Can you work these out from the model? Positions are in its coordinate system, mm. A direction names the side the tool comes from. Coordinates: 2 decimals unless noted, no trailing zeros. Order: outer loops, then holes, each group sorted by start corner. A loop starts at its lowest first (then second) coordinate and runs counter-clockwise, first axis right, second up. Notation, with made-up numbers: (16.25, -8) - (49.25, -8) arc R21 cw to (49.25, 2) - close; hole circle Ø10 at (6, -29.75). An arc over 180 degrees is marked (long way). Return JSON: item names as keys, results as strings. Group by question number.
1) If we mould it in two halves opening along X, with no side actions, what happens to faces 4 (the face through (-29.599, 36.454, 1.521)), 5 (the face through (42.196, -44.527, 0.171)), 6 (the face through (34.93, -37.55, 0.65)), 7 (the face through (-39.64, 36.85, 2.83))? For each: pulls with the +X half, pulls with the -X half, needs draft (parallel to the pull), parting line crosses it, or undercut.
2) Imagine slicing it at A-A (y = -17.5). Write out the boundary of the cut face in (x, z).
3) For pin 1 Ø0.8 at (x, z) = (2, 0.5) entering from -Y; pin 2 Ø3 at (x, y) = (-40.72, -34.34) entering from +Z, each with a flat end and sliding along its axis, tell me the tip position at first contact or that it passes through.
4) Which directions (+Z, -Z, +X, -X, +Y, -Y) give clear straight access to the entire face, cutting with the end or side of a thin tool? Please do faces 1 (the face through (-32.92, 30.446, 1.792)), 2 (the face through (34.997, 29.81, 0.645)), 3 (the face through (35.079, 29.89, 0.185)).
5) Imagine slicing it at B-B (x = 19). Write out the boundary of the cut face in (y, z), and give its area (3 significant figures).
6) If I drill on line 1 along Y through (x, z) = (1, 0.65); line 2 along X through (y, z) = (-6.5, 2.4); line 3 along Y through (x, z) = (28.5, 1.5), over which ranges is the centre line in solid material (lowest first)?
```python
from build123d import *

# Parameters (mm, degrees)
SKETCH2_R           = 1.25
BOSS_EXTRUDE1_DEPTH = 3
CHAMFER1_SIZE       = 2
CHAMFER2_SIZE       = 0.6
CHAMFER3_SIZE       = 0.3
SKETCH3_R           = 1.75
CUT_EXTRUDE1_DEPTH  = 4


with BuildPart() as part:
    # Sketch2 → Boss-Extrude1 (new body)
    with BuildSketch(Plane.XY):
        with BuildLine():
            Line((-44.219607843, -34.337254902), (-44.219607843, 26.662745098))
            ThreePointArc((-44.219607843, 26.662745098), (-39.826209561, 37.269346816), (-29.219607843, 41.662745098))
            Line((-29.219607843, 41.662745098), (31.780392157, 41.662745098))
            ThreePointArc((31.780392157, 41.662745098), (42.386993875, 37.269346816), (46.780392157, 26.662745098))
            Line((46.780392157, 26.662745098), (46.780392157, -34.337254902))
            ThreePointArc((46.780392157, -34.337254902), (42.386993875, -44.94385662), (31.780392157, -49.337254902))
            Line((31.780392157, -49.337254902), (-29.219607843, -49.337254902))
            ThreePointArc((-29.219607843, -49.337254902), (-39.826209561, -44.94385662), (-44.219607843, -34.337254902))
        make_face()
        with Locations((43.280392157, -34.337254902)):
            Circle(SKETCH2_R, mode=Mode.SUBTRACT)
        with Locations((31.780392157, 38.162745098)):
            Circle(SKETCH2_R, mode=Mode.SUBTRACT)
        with Locations((-29.219607843, 38.162745098)):
            Circle(SKETCH2_R, mode=Mode.SUBTRACT)
        with Locations((-40.719607843, -34.337254902)):
            Circle(SKETCH2_R, mode=Mode.SUBTRACT)
        with BuildLine():
            ThreePointArc((-29.219607843, 31.162745098), (-32.401588358, 29.844725613), (-33.719607843, 26.662745098))
            Line((-33.719607843, 26.662745098), (-33.719607843, -34.337254902))
            ThreePointArc((-33.719607843, -34.337254902), (-32.401588358, -37.519235417), (-29.219607843, -38.837254902))
            Line((-29.219607843, -38.837254902), (31.780392157, -38.837254902))
            ThreePointArc((31.780392157, -38.837254902), (34.962372672, -37.519235417), (36.280392157, -34.337254902))
            Line((36.280392157, -34.337254902), (36.280392157, 26.662745098))
            ThreePointArc((36.280392157, 26.662745098), (34.962372672, 29.844725613), (31.780392157, 31.162745098))
            Line((31.780392157, 31.162745098), (-29.219607843, 31.162745098))
        make_face(mode=Mode.SUBTRACT)
    extrude(amount=BOSS_EXTRUDE1_DEPTH)

    # Chamfer1
    chamfer1_edges = [part.edges().sort_by_distance(p)[0] for p in [
        (-32.401588358, 29.844725613, 3),
        (1.280392157, 31.162745098, 3),
        (34.962372672, 29.844725613, 3),
        (36.280392157, -3.837254902, 3),
        (34.962372672, -37.519235417, 3),
        (1.280392157, -38.837254902, 3),
        (-32.401588358, -37.519235417, 3),
        (-33.719607843, -3.837254902, 3),
    ]]
    chamfer(chamfer1_edges, length=CHAMFER1_SIZE)

    # Chamfer2
    chamfer2_edges = [part.edges().sort_by_distance(p)[0] for p in [
        (1.280392157, 41.662745098, 3),
        (-39.826209561, 37.269346816, 3),
        (-39.826209561, 37.269346816, 0),
        (1.280392157, 41.662745098, 0),
        (42.386993875, 37.269346816, 0),
        (46.780392157, -3.837254902, 0),
        (42.386993875, -44.94385662, 0),
        (1.280392157, -49.337254902, 0),
        (-39.826209561, -44.94385662, 0),
        (-44.219607843, -3.837254902, 0),
        (-44.219607843, -3.837254902, 3),
        (-39.826209561, -44.94385662, 3),
        (1.280392157, -49.337254902, 3),
        (42.386993875, -44.94385662, 3),
        (46.780392157, -3.837254902, 3),
        (42.386993875, 37.269346816, 3),
    ]]
    chamfer(chamfer2_edges, length=CHAMFER2_SIZE)

    # Chamfer3
    chamfer3_edges = [part.edges().sort_by_distance(p)[0] for p in [
        (-33.719607843, -3.837254902, 0),
        (-32.401588358, -37.519235417, 0),
        (1.280392157, -38.837254902, 0),
        (34.962372672, -37.519235417, 0),
        (36.280392157, -3.837254902, 0),
        (34.962372672, 29.844725613, 0),
        (1.280392157, 31.162745098, 0),
        (-32.401588358, 29.844725613, 0),
    ]]
    chamfer(chamfer3_edges, length=CHAMFER3_SIZE)

    # Sketch3 → Cut-Extrude1 (cut, through all)
    with BuildSketch(Plane.XY.offset(3)):
        with Locations((-29.219607843, 38.162745098)):
            Circle(SKETCH3_R)
        with Locations((31.780392157, 38.162745098)):
            Circle(SKETCH3_R)
        with Locations((-40.719607843, -34.337254902)):
            Circle(SKETCH3_R)
        with Locations((43.280392157, -34.337254902)):
            Circle(SKETCH3_R)
    extrude(amount=-CUT_EXTRUDE1_DEPTH, mode=Mode.SUBTRACT)


solid = part.part
```
Calculated:
{
 "1": {"face 4": "undercut", "face 5": "pulls with the +X half", "face 6": "undercut", "face 7": "pulls with the -X half"},
 "2": {"outline": "(-44.22, 0.6) - (-43.62, 0) - (-34.02, 0) - (-33.72, 0.3) - (-33.72, 1) - (-35.72, 3) - (-43.62, 3) - (-44.22, 2.4) - close; (36.28, 0.3) - (36.58, 0) - (46.18, 0) - (46.78, 0.6) - (46.78, 2.4) - (46.18, 3) - (38.28, 3) - (36.28, 1) - close"},
 "3": {"pin 1": "y = -49.34", "pin 2": "through"},
 "4": {"face 1": "+Z", "face 2": "+Z, -Z", "face 3": "-Z"},
 "5": {"outline": "(-49.34, 0.6) - (-48.74, 0) - (-39.14, 0) - (-38.84, 0.3) - (-38.84, 1) - (-40.84, 3) - (-48.74, 3) - (-49.34, 2.4) - close; (31.16, 0.3) - (31.46, 0) - (41.06, 0) - (41.66, 0.6) - (41.66, 2.4) - (41.06, 3) - (33.16, 3) - (31.16, 1) - close", "area": "58.2 mm2"},
 "6": {"line 1": "-49.34 to -38.84, 31.16 to 41.66", "line 2": "-44.22 to -35.12, 37.68 to 46.78", "line 3": "-49.34 to -39.34, 31.66 to 41.66"}
}
